The drawing under review shows one solid part. Ordinate dimensions are in mm from its lowest x, y, z. Coordinates: 2 decimals unless noted, no trailing zeros. Order: outer loops, then holes, each group sorted by start corner. A loop starts at its lowest first (then second) coordinate and runs counter-clockwise, first axis right, second up. Notation, with made-up numbers: (66, 24) -> (87, 24) arc R26 cw to (87, 58) -> close; hole circle Ø10 at (27, -36). An arc over 180 degrees is marked (long way). Put each result on its own line as item: value.
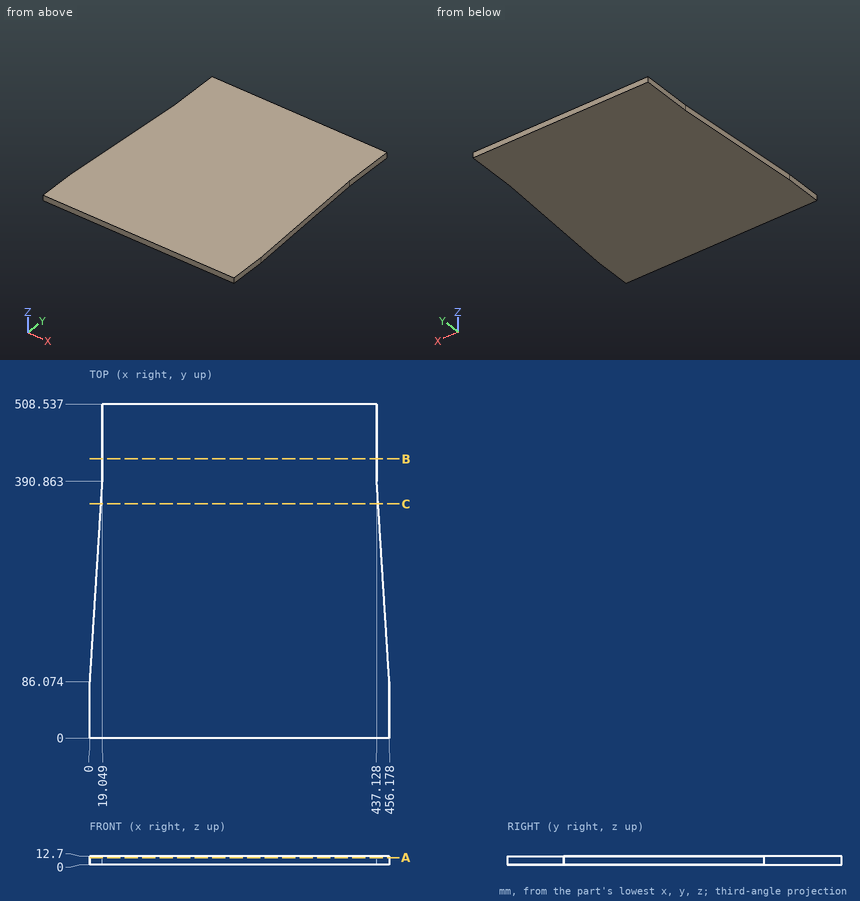
Item 1: For pin 1 Ø5 at (x, z) = (240.5, 7) entering from -Y; pin 2 Ø5 at (y, z) = (255, 11) entering from +X; pin 3 Ø1 at (y, z) = (108.5, 3.5) entering from +X; pin 4 Ø1 at (y, z) = (181, 9.5) entering from +X, all flat-tipped, find the tip position at first contact; note any pin that passes through.
Answers below:
pin 1: y = 0
pin 2: x = 445.78
pin 3: x = 454.81
pin 4: x = 450.28
Item 2: For line 1 (X direction, y = 457.5, z = 3.75); line 2 (X direction, y = 163, z = 1), list the stretches that pass through material, from the lowest coordinate up. Write a range as from..to.
Answers below:
line 1: 19.05..437.13
line 2: 4.81..451.37
Item 3: Consider section B-B on y = 425. Write out the cut boundary in (x, z).
Answers below:
outline: (19.05, 0) -> (437.13, 0) -> (437.13, 12.7) -> (19.05, 12.7) -> close
Item 4: Consider section C-C on y = 356.5. Write out the cut boundary in (x, z) (1 decimal).
Answers below:
outline: (16.9, 0) -> (439.3, 0) -> (439.3, 12.7) -> (16.9, 12.7) -> close
Item 5: Consider section A-A on z = 10.5. Write out the cut boundary in (x, y).
Answers below:
outline: (0, 0) -> (456.18, 0) -> (456.18, 86.07) -> (437.13, 390.86) -> (437.13, 508.54) -> (19.05, 508.54) -> (19.05, 390.86) -> (0, 86.07) -> close
